Work out the finished part from the listing and answer in its coordinate system (mm). Face numbers are marked on the shaded views. A direction names the side the tool comes from. Give positions to 0.01 mm unless a question says otherwise; leave off trailing zeros. Order: outer loops, then holes, each group sorted by start corner. A loop starts at its lowest first (then second) coordinate and runs counter-clockwise, first axis right, second up.
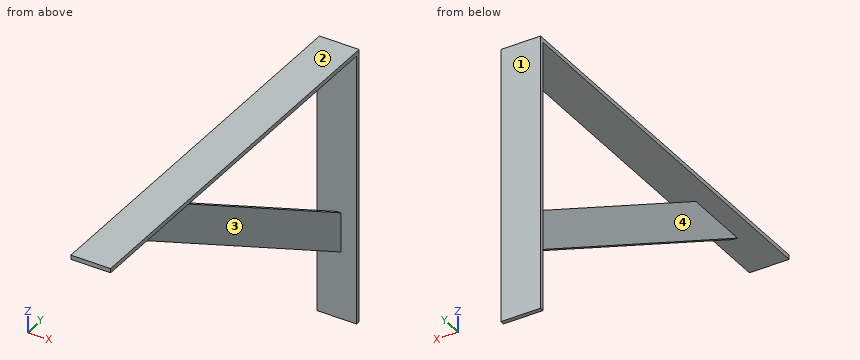
```python
from build123d import *

# Parameters (mm, degrees)
F0_W     = 29.464
F0_H     = 296.926
F1_DEPTH = 3.175
F2_W     = 29.464
F2_H     = 204.978
F3_DEPTH = 3.175
F6_DEPTH = 3.175


with BuildPart() as f1:
    # F0 (on Top) → F1 (new body)
    with BuildSketch(Plane.XY):
        Rectangle(F0_W, F0_H)
    extrude(amount=F1_DEPTH)

    # F2 (on face) → F3 (join)
    with BuildSketch(Plane(origin=(0, 148.463, 0), x_dir=(-1, 0, 0), z_dir=(0, 1, 0))):
        with Locations((0, -99.314)):
            Rectangle(F2_W, F2_H)
    extrude(amount=-F3_DEPTH)

    # F5 (on offset) → F6 (join)
    with BuildSketch(Plane.YZ.offset(3.175)):
        Polygon((145.288, -151.575044), (145.288, -122.111044), (-60.823944, 0), (-110.556401, 0), align=None)
    extrude(amount=-F6_DEPTH)


solid = f1.part
```
1. The part is cut by section C-C (x = 7.25). Write down the section's boundary in (y, z) (3 decimals).
Findings below:
outline: (-148.463, 0) - (145.288, 0) - (145.288, -201.803) - (148.463, -201.803) - (148.463, 3.175) - (-148.463, 3.175) - close
2. Given P1, Ø14.5, axis at x = 2.5, y = 26.5, coming from the -Z side; P2, Ø9, axis at x = 2, z = -119.5, coming from the -Y side; P3, Ø1.5, axis at x = -3.5, z = -50.5, coming from the -Y side, each flat-ended and moving along its own axis, determine where each tip first touches the part or whether it passes through.
Findings below:
P1: stops at z = -85.49
P2: stops at y = 83.55
P3: stops at y = 145.29
3. Straight lines are drawn through the part: probe 1 along Z at (x, y) = (4.25, 91.5) (3 decimals); probe 2 along Y at (x, z) = (-6.75, -140). For each, find the intervals that lie inside material, in ascending order.
Findings below:
probe 1: z = 0 to 3.175
probe 2: y = 145.29 to 148.46
4. Which of the six approach directions +Z, -Z, +X, -X, +Y, -Y give full straight-line access (tool end or side, diameter ignored) to the marked faces 3 and 4?
Findings below:
face 3: -Z, +X, -Y
face 4: -Z, -X, -Y
5. The part is cut by section A-A (z = -54.5). Write down the section's boundary in (x, y) (3 decimals).
Findings below:
outline: (-14.732, 145.288) - (14.732, 145.288) - (14.732, 148.463) - (-14.732, 148.463) - close; (0, -18.566) - (3.175, -18.566) - (3.175, 31.167) - (0, 31.167) - close
6. The mould has two halves that part along Z. Classify the marked faces 1 and 2: pulls with the +Z half, pulls with the -Z half, needs draft (parallel to the pull), parting line crosses it, or undercut.
Findings below:
face 1: needs draft
face 2: pulls with the +Z half
7. The part is cut by section B-B (y = 56). Write down the section's boundary in (x, z) (3 decimals), then the cut area to 3 significant figures.
Findings below:
outline: (-14.732, 0) - (14.732, 0) - (14.732, 3.175) - (-14.732, 3.175) - close; (0, -98.676) - (3.175, -98.676) - (3.175, -69.212) - (0, -69.212) - close
area: 187 mm2
8. The part is cut by section D-D (y = -78). Write down the section's boundary in (x, z) (3 decimals).
Findings below:
outline: (-14.732, 0) - (0, 0) - (0, -19.288) - (3.175, -19.288) - (3.175, 0) - (14.732, 0) - (14.732, 3.175) - (-14.732, 3.175) - close
